```python
from build123d import *

# Parameters (mm, degrees)
SKETCH_1_R          = 11.5
SKETCH_1_R_2        = 1.6
SKETCH_1_R_3        = 1.05
SKETCH_1_R_4        = 2.6
EXTRUDE_1_DEPTH     = 4.7
SKETCH_2_R          = 2
SKETCH_2_R_2        = 6
CUT_EXTRUDE_1_DEPTH = 0.5
SKETCH_5_R          = 2
CUT_EXTRUDE_2_DEPTH = 2
FILLET_1_R          = 2


with BuildPart() as part:
    # 草图1 → 凸台-拉伸1 (new body)
    with BuildSketch(Plane.XY):
        Polygon((0, 0), (135, 0), (135, -52), (0, -52), (-8, -52), (-8, -28), (-2, -28), (-2, 0), align=None)
        with Locations((13, -15)):
            Circle(SKETCH_1_R, mode=Mode.SUBTRACT)
        with Locations((1.5, -3.5)):
            Circle(SKETCH_1_R_2, mode=Mode.SUBTRACT)
        with Locations((24.5, -3.5)):
            Circle(SKETCH_1_R_2, mode=Mode.SUBTRACT)
        with Locations((1.5, -26.5)):
            Circle(SKETCH_1_R_2, mode=Mode.SUBTRACT)
        with Locations((24.5, -26.5)):
            Circle(SKETCH_1_R_2, mode=Mode.SUBTRACT)
        with Locations((32.5, -10)):
            Circle(SKETCH_1_R_3, mode=Mode.SUBTRACT)
        with Locations((44.5, -10)):
            Circle(SKETCH_1_R_3, mode=Mode.SUBTRACT)
        with Locations((32.5, -18)):
            Circle(SKETCH_1_R_3, mode=Mode.SUBTRACT)
        with Locations((44.5, -18)):
            Circle(SKETCH_1_R_3, mode=Mode.SUBTRACT)
        with Locations((117.5, -10)):
            Circle(SKETCH_1_R_3, mode=Mode.SUBTRACT)
        with Locations((129.5, -10)):
            Circle(SKETCH_1_R_3, mode=Mode.SUBTRACT)
        with Locations((117.5, -18)):
            Circle(SKETCH_1_R_3, mode=Mode.SUBTRACT)
        with Locations((129.5, -18)):
            Circle(SKETCH_1_R_3, mode=Mode.SUBTRACT)
        with Locations((-0.75, -33)):
            Circle(SKETCH_1_R_3, mode=Mode.SUBTRACT)
        with Locations((7.25, -33)):
            Circle(SKETCH_1_R_3, mode=Mode.SUBTRACT)
        with Locations((-0.75, -45)):
            Circle(SKETCH_1_R_3, mode=Mode.SUBTRACT)
        with Locations((7.25, -45)):
            Circle(SKETCH_1_R_3, mode=Mode.SUBTRACT)
        with Locations((29.25, -33)):
            Circle(SKETCH_1_R_3, mode=Mode.SUBTRACT)
        with Locations((37.25, -33)):
            Circle(SKETCH_1_R_3, mode=Mode.SUBTRACT)
        with Locations((37.25, -45)):
            Circle(SKETCH_1_R_3, mode=Mode.SUBTRACT)
        with Locations((29.25, -45)):
            Circle(SKETCH_1_R_3, mode=Mode.SUBTRACT)
        with Locations((117.5, -40)):
            Circle(SKETCH_1_R_3, mode=Mode.SUBTRACT)
        with Locations((129.5, -40)):
            Circle(SKETCH_1_R_3, mode=Mode.SUBTRACT)
        with Locations((117.5, -48)):
            Circle(SKETCH_1_R_3, mode=Mode.SUBTRACT)
        with Locations((129.5, -48)):
            Circle(SKETCH_1_R_3, mode=Mode.SUBTRACT)
        with Locations((55, -28)):
            Circle(SKETCH_1_R_4, mode=Mode.SUBTRACT)
        with Locations((55, -47)):
            Circle(SKETCH_1_R_4, mode=Mode.SUBTRACT)
        with Locations((77.25, -33)):
            Circle(SKETCH_1_R_3, mode=Mode.SUBTRACT)
        with Locations((77.25, -45)):
            Circle(SKETCH_1_R_3, mode=Mode.SUBTRACT)
        with Locations((69.25, -45)):
            Circle(SKETCH_1_R_3, mode=Mode.SUBTRACT)
        with Locations((69.25, -33)):
            Circle(SKETCH_1_R_3, mode=Mode.SUBTRACT)
        with Locations((55, -9)):
            Circle(SKETCH_1_R_4, mode=Mode.SUBTRACT)
    extrude(amount=EXTRUDE_1_DEPTH)

    # 草图2 → 切除-拉伸1 (cut)
    with BuildSketch(Plane.XY.offset(4.7)):
        with Locations((32.5, -10)):
            Circle(SKETCH_2_R)
        with Locations((44.5, -10)):
            Circle(SKETCH_2_R)
        with Locations((32.5, -18)):
            Circle(SKETCH_2_R)
        with Locations((44.5, -18)):
            Circle(SKETCH_2_R)
        with Locations((117.5, -10)):
            Circle(SKETCH_2_R)
        with Locations((129.5, -10)):
            Circle(SKETCH_2_R)
        with Locations((117.5, -18)):
            Circle(SKETCH_2_R)
        with Locations((129.5, -18)):
            Circle(SKETCH_2_R)
        with Locations((117.5, -40)):
            Circle(SKETCH_2_R)
        with Locations((129.5, -40)):
            Circle(SKETCH_2_R)
        with Locations((117.5, -48)):
            Circle(SKETCH_2_R)
        with Locations((55, -28)):
            Circle(SKETCH_2_R_2)
        with Locations((129.5, -48)):
            Circle(SKETCH_2_R)
        with Locations((55, -47)):
            Circle(SKETCH_2_R_2)
        with Locations((55, -9)):
            Circle(SKETCH_2_R_2)
    extrude(amount=-CUT_EXTRUDE_1_DEPTH, mode=Mode.SUBTRACT)

    # 草图5 → 切除-拉伸2 (cut)
    with BuildSketch(Plane(origin=(0, 0, 0), x_dir=(-1, 0, 0), z_dir=(0, 0, -1))):
        with Locations((-37.25, -33)):
            Circle(SKETCH_5_R)
        with Locations((-29.25, -33)):
            Circle(SKETCH_5_R)
        with Locations((-37.25, -45)):
            Circle(SKETCH_5_R)
        with Locations((-29.25, -45)):
            Circle(SKETCH_5_R)
        with Locations((-7.25, -33)):
            Circle(SKETCH_5_R)
        with Locations((0.75, -33)):
            Circle(SKETCH_5_R)
        with Locations((-7.25, -45)):
            Circle(SKETCH_5_R)
        with Locations((0.75, -45)):
            Circle(SKETCH_5_R)
        with Locations((-69.25, -33)):
            Circle(SKETCH_5_R)
        with Locations((-69.25, -45)):
            Circle(SKETCH_5_R)
        with Locations((-77.25, -45)):
            Circle(SKETCH_5_R)
        with Locations((-77.25, -33)):
            Circle(SKETCH_5_R)
    extrude(amount=-CUT_EXTRUDE_2_DEPTH, mode=Mode.SUBTRACT)

    # 圆角1
    fillet_1_edges = [part.edges().sort_by_distance(p)[0] for p in [
        (-2, -28, 2.35),
        (-2, 0, 2.35),
    ]]
    fillet(fillet_1_edges, radius=FILLET_1_R)


solid = part.part
```
Design review of the part built by this model. Coordinates are the model's own, in mm. A direction names the side the tool comes from. Round coordinates to 2 decimals unless told otherwise and drop trailing zeros. Write each loop counter-clockwise with the first axis right and the second up, starting at its lowest first coordinate (ties: lowest second). Pieces come first, ordered by that corner, then holes. Notation, with made-up numbers: (39.5, 3) -> (92.5, 3) arc R18 cw to (92.5, 16) -> close; hole circle Ø9 at (35, 70.25). An arc over 180 degrees is marked (long way). Write item = value, one per line. Start each with the question number.
1) Take a section at B-B, the plane z = 0.9. Count the separate pieces of the cut face and the enclosed holes in it, plus the area to 3 significant figures.
2) Clearance check with flat-ended pins moving along their axes: pin 1 (1.2 mm diameter, centred on x = 29.5, y = -32, fed in from -Z); pin 2 (1.2 mm diameter, centred on x = 32, y = -17.5, fed in from +Z). State where each tip first meets the part, or that it passes through.
3) Take a section at A-A, the plane x = 13. State the section outline as (y, z) points.
4) Wall thickness on probe 1 along Y at (x, z) = (55, 4.55); probe 2 along Y at (x, z) = (69.25, 3.4); probe 3 along X at (y, z) = (-40, 3.35): over which ranges is each line inside the solid? List them lowest first. Write a range as from..to.
5) Mouldability with a two-part tool opening along X and no side actions: class faces 1 (the face through (-6, -28, 2)), 2 (the face through (7.684, -46.952, 0.986)), 3 (the face through (45.4, -10.9, 4.2)), 4 (the face through (-2, -14, 2)) as +X half, -X half, draft (parallel to the pull), parting line (faces both ways), or undercut.
6) Tool access review of faces 5 (the face through (33.4, -18.9, 4.2)), 6 (the face through (65, -26, 0)), 7 (the face through (76.327, -34.774, 0.986)): name each direction out of +Z, -Z, +X, -X, +Y, -Y from which nothing blocks a thin tool from reaching the whole face with its end or side.
Results list:
q1.separate_pieces = 1
q1.enclosed_holes = 32
q1.area = 6,560 mm²
q2.pin_1 = 2
q2.pin_2 = 4.2
q3.outline = (-52, 0) -> (-26.5, 0) -> (-26.5, 4.7) -> (-52, 4.7) -> close; (-3.5, 0) -> (0, 0) -> (0, 4.7) -> (-3.5, 4.7) -> close
q4.probe_1 = -41..-34, -22..-15, -3..0
q4.probe_2 = -52..-46.05, -43.95..-34.05, -31.95..0
q4.probe_3 = -8..116.45, 118.55..128.45, 130.55..135
q5.face_1 = draft
q5.face_2 = undercut
q5.face_3 = undercut
q5.face_4 = -X half
q6.face_5 = +Z
q6.face_6 = -Z, +X, -X, +Y, -Y
q6.face_7 = -Z
